Design review of the part built by this model. Coordinates are the model's own, in mm. A direction names the side the tool comes from. Coordinates: 2 decimals unless noted, no trailing zeros. Write each loop counter-clockwise with the first axis right and the second up, starting at its lowest first coordinate (ties: lowest second). Pieces come first, ordered by that corner, then holes. Notation, with made-up numbers: (5, -33.75) - (51, -33.75) arc R12 ccw to (51, -10.75) - close; hole circle Ø11 at (-39.5, 3). An arc over 180 degrees is marked (long way). One line per item, written item: value.
Autodesk Inventor part; units mm, degrees
ref_plane "YZ Plane" through (0, 0, 0) normal (1, 0, 0) x (0, 1, 0)
ref_plane "XZ Plane" through (0, 0, 0) normal (0, 1, 0) x (-1, 0, 0)
ref_plane "XY Plane" through (0, 0, 0) normal (0, 0, 1) x (1, 0, 0)
sketch "Sketch1" plane through (0, 0, 0) normal (0, 1, 0) x (-1, 0, 0)
  line L0 (10, -16) -> (-10, -16)
  line L1 (-10, -16) -> (-10, 16)
  line L2 (-10, 16) -> (10, 16)
  line L3 (10, 16) -> (10, -16)
  point P0 (0, 0)
  point P1 (0, -16)
  point P2 (10, 0)
  dimension "d0" = 20
  dimension "d1" = 32
extrude "Extrusion1" add sketch "Sketch1" along normal blind 1.1
sketch "Sketch2" plane through (0, 1.1, 0) normal (0, 1, 0) x (1, 0, 0)
  circle A0 centre (-7.5, -13.5) radius 1.5
  line L0 (-10, -16) -> (10, -16)
  line L1 (-10, 16) -> (-10, -16)
  line L2 (-10, 0) -> (10, 0) construction
  line L3 (0, -16) -> (0, 16)
  circle A1 centre (-7.5, 13.5) radius 1.5
  circle A2 centre (7.5, -13.5) radius 1.5
  circle A3 centre (7.5, 13.5) radius 1.5
  point P0 (0, 0)
  dimension "d4" = 3
  dimension "d5" = 2.5
  dimension "d6" = 2.5
extrude "Extrusion2" cut sketch "Sketch2" against normal through all
sketch "Sketch3" plane through (0, 1.1, 0) normal (0, 1, 0) x (1, 0, 0)
  circle A0 centre (0, -6) radius 9
  line L0 (-10, -16) -> (10, -16)
  point P0 (0, 0)
  dimension "d9" = 18
  dimension "d10" = 10
extrude "Extrusion3" add sketch "Sketch3" along normal blind 5
fillet "Fillet1" radius 0.5 1 edges at (-9, 6.1, 6)
sketch "Sketch4" plane through (0, 0, 0) normal (1, 0, 0) x (0, 1, 0)
  line L0 (1.1, 15) -> (5.6, 15) construction
  line L1 (1.1, 15) -> (1.1, 12) construction
  arc A0 (6.1, 14.5) -> (5.6, 15) centre (5.6, 14.5) ccw
  line L2 (1.1, 15) -> (1.1, 12.0001)
  line L3 (1.1, 15) -> (1.6, 15)
  line L4 (1.1, 15) -> (1.1, 14.5)
  arc A1 (1.6, 15) -> (1.1, 14.5) centre (1.6, 14.5) ccw
  line L5 (6.1, 6) -> (3.5731, 6) construction
  line L6 (6.1, 14.5) -> (6.1, -2.5) construction
  point P0 (0, 0)
  point P1 (1.1, 6)
  dimension "d17" = 0.5
  dimension "d18" = 0.5
revolve "Revolution1" cut sketch "Sketch4" angle 360 about axis through (0, 6.1, 6) along (0, -1, 0)
sketch "Sketch5" plane through (0, 0, 0) normal (1, 0, 0) x (0, 1, 0)
  line L0 (13.274, 6) -> (6.1, 6)
  line L1 (6.1, 14.5) -> (6.1, -2.5)
  arc A0 (6.1, 14.166) -> (6.9626, 13.1755) centre (7.1, 14.166) ccw
  line L2 (13.274, 12.3) -> (13.274, 6)
  line L3 (13.274, 12.3) -> (6.9626, 13.1755)
  line L4 (6.1, 14.166) -> (6.1, 6)
  line L5 (14.9992, 10.319) -> (14.9992, 6)
  line L6 (13.274, 6) -> (14.9992, 6)
  arc A1 (14.9992, 10.319) -> (13.274, 12.3) centre (12.9992, 10.319) ccw
  point P0 (0, 0)
  point P1 (13.274, 10.9657)
  dimension "d20" = 2
  dimension "d21" = 0.334
  dimension "d22" = 7.174
  dimension "d23" = 6.3
  dimension "d35" = 4
revolve "Revolution2" add sketch "Sketch5" angle 360 about axis through (0, 13.274, 6) along (0, -1, 0)
sketch "Sketch6" plane through (0, 0, 0) normal (0, -1, 0) x (1, 0, 0)
  circle A0 centre (0, 6) radius 7.166
  circle A1 centre (0, 6) radius 5 construction
  circle A2 centre (5, 6) radius 0.5
  circle A3 centre (4.3301, 8.5) radius 0.5
  circle A4 centre (2.5, 10.3301) radius 0.5
  circle A5 centre (0, 11) radius 0.5
  circle A6 centre (-2.5, 10.3301) radius 0.5
  circle A7 centre (-4.3301, 8.5) radius 0.5
  circle A8 centre (-5, 6) radius 0.5
  circle A9 centre (-4.3301, 3.5) radius 0.5
  circle A10 centre (-2.5, 1.6699) radius 0.5
  circle A11 centre (0, 1) radius 0.5
  circle A12 centre (2.5, 1.6699) radius 0.5
  circle A13 centre (4.3301, 3.5) radius 0.5
  point P0 (0, 0)
  dimension "d27" = 10
  dimension "d28" = 1
  dimension "d31" = 360
extrude "Extrusion4" add sketch "Sketch6" along normal blind 5 contours A2 | A3 | A7 | A8 | A9 | A13
sketch "Sketch7" plane through (0, 0, 0) normal (0, -1, 0) x (1, 0, 0)
  line L0 (5, -11) -> (-5, -11)
  line L1 (-5, -11) -> (-5, -13.5)
  line L2 (-5, -13.5) -> (5, -13.5)
  line L3 (5, -13.5) -> (5, -11)
  line L4 (-10, -16) -> (10, -16)
  point P0 (0, 0)
  point P1 (0, -13.5)
  dimension "d36" = 10
  dimension "d37" = 2.5
  dimension "d38" = 2.5
extrude "Extrusion5" add sketch "Sketch7" along normal blind 2.5
sketch "Sketch8" plane through (0, -2.5, 0) normal (0, -1, 0) x (1, 0, 0)
  line L0 (4.2, -12.7) -> (3.3, -12.7)
  line L1 (3.3, -12.7) -> (3.3, -11.8)
  line L2 (3.3, -11.8) -> (4.2, -11.8)
  line L3 (4.2, -11.8) -> (4.2, -12.7)
  line L4 (5, -13.5) -> (5, -11)
  line L5 (5, -11) -> (-5, -11)
  line L6 (-5, -11) -> (-5, -13.5)
  line L7 (-5, -13.5) -> (5, -13.5)
  line L8 (5, -13.5) -> (5, -11)
  line L9 (1.7, -12.7) -> (0.8, -12.7)
  line L10 (1.7, -11.8) -> (1.7, -12.7)
  line L11 (0.8, -12.7) -> (0.8, -11.8)
  line L12 (0.8, -11.8) -> (1.7, -11.8)
  line L13 (-0.8, -12.7) -> (-1.7, -12.7)
  line L14 (-0.8, -11.8) -> (-0.8, -12.7)
  line L15 (-1.7, -12.7) -> (-1.7, -11.8)
  line L16 (-1.7, -11.8) -> (-0.8, -11.8)
  line L17 (-3.3, -12.7) -> (-4.2, -12.7)
  line L18 (-3.3, -11.8) -> (-3.3, -12.7)
  line L19 (-4.2, -12.7) -> (-4.2, -11.8)
  line L20 (-4.2, -11.8) -> (-3.3, -11.8)
  point P0 (0, 0)
  point P1 (5, -12.25)
  point P2 (4.2, -12.25)
  point P3 (1.7, -12.25)
  point P4 (-0.8, -12.25)
  point P5 (-3.3, -12.25)
  dimension "d41" = 0.9
  dimension "d42" = 0.9
  dimension "d43" = 0.8
  dimension "d46" = 2.5
extrude "Extrusion6" add sketch "Sketch8" along normal blind 2 contours L0 L1 L2 L3 | L9 L11 L12 L10 | L13 L15 L16 L14 | L17 L19 L20 L18
sketch "Sketch9" plane through (4.2, -2.5, -12.7) normal (0, 0, -1) x (-1, 0, 0)
  line L0 (0, 0) -> (0.9, 0)
  line L1 (0, 0) -> (0, -2)
  line L2 (0.9, -2) -> (0, -2)
  line L3 (0.9, 0) -> (0.9, -2)
  line L4 (0.9, -1.1) -> (0, -1.1)
  point P0 (4.2, 2.5)
  dimension "d53" = 0.9
  dimension "d54" = 0.9
extrude "Extrusion7" add sketch "Sketch9" along normal blind 8 contours L4 L3 L2 L1
chamfer "Chamfer1" distance 0.3 angle 45 4 edges at (4.2, -4.05, -20.7) (3.75, -4.5, -20.7) (3.3, -4.05, -20.7) (3.75, -3.6, -20.7)
pattern_linear "Rectangular Pattern1" count 4 spacing 2.5 along (-1, 0, 0) of "Extrusion7", "Chamfer1"
equation "\"d53\" = d54"
properties part number "MQ_New" material "Steel, Mild, Welded"
1. Insertion check: pin 1 Ø6 at (y, z) = (5, -7) entering from +X; pin 2 Ø2 at (y, z) = (-3.5, -15) entering from +X; pin 3 Ø4 at (x, y) = (7, 1.5) entering from -Z; pin 4 Ø0.7 at (x, y) = (3.5, -3) entering from -Z. Each pin has a flat end and moves straight along its axis. Give the tip position at first contact, or say it passes through.
Answer block:
pin 1: passes through
pin 2: stops at x = 4.2
pin 3: stops at z = -16
pin 4: stops at z = -12.7
2. For faces 1 (the face through (0, -1, -13.5)), 2 (the face through (-1, -3, -11.8)), 3 (the face through (4.3, -2.5, 3)), 4 (the face through (-5, -1, -12)), 5 (the face through (5, -1, -12)), list the 3-axis set-ups (+Z, -Z, +X, -X, +Y, -Y) from which the entire face can be reached by the end or side of a thin tool; tool diameter is ignored.
Answer block:
face 1: -Z, +X, -X
face 2: +Z, +X, -X, -Y
face 3: -Y
face 4: -Z, -X, -Y
face 5: -Z, +X, -Y
3. Consider section B-B, the plane z = -17.5. Write out the cut boundary in (x, y).
Answer block:
outline: (-4.2, -4.5) - (-3.3, -4.5) - (-3.3, -3.6) - (-4.2, -3.6) - close; (-1.7, -4.5) - (-0.8, -4.5) - (-0.8, -3.6) - (-1.7, -3.6) - close; (0.8, -4.5) - (1.7, -4.5) - (1.7, -3.6) - (0.8, -3.6) - close; (3.3, -4.5) - (4.2, -4.5) - (4.2, -3.6) - (3.3, -3.6) - close
4. Consider section D-D, the plane y = 4. Write out the cut boundary in (x, z).
Answer block:
outline: circle Ø18 at (0, 6)
5. Wall thickness on line 1 along X through (y, z) = (0.4, -13.5); line 2 along Z through (x, y) = (7.5, 0.35); line 3 along Z through (x, y) = (6.25, 1): over which ranges is each line inside the solid? List them lowest first.
Answer block:
line 1: x = -10 to -9, -6 to 6, 9 to 10
line 2: z = -16 to -15, -12 to 12, 15 to 16
line 3: z = -16 to -14.33, -12.67 to 12.67, 14.33 to 16
6. Mouldability with a two-part tool opening along X and no side actions: class faces 6 (the face through (0, -1, -11)), 7 (the face through (-2, 10.78, 12.34)), 8 (the face through (1.7, -4, -16)) as released by +X, released by -X, zero draft, split by the parting line, or undercut.
Answer block:
face 6: zero draft
face 7: split by the parting line
face 8: undercut
7. Consider section A-A, the plane y = 0.5. Write out the cut boundary in (x, z), then the cut area to 3 significant figures.
Answer block:
outline: (-10, -16) - (10, -16) - (10, 16) - (-10, 16) - close; hole circle Ø3 at (-7.5, -13.5); hole circle Ø3 at (-7.5, 13.5); hole circle Ø3 at (7.5, -13.5); hole circle Ø3 at (7.5, 13.5)
area: 612 mm^2
8. Consider section C-C, the plane z = 6. Write out the cut boundary in (x, y), then the cut area to 3 significant figures.
Answer block:
outline: (-10, 0) - (-5.5, 0) - (-5.5, -5) - (-4.5, -5) - (-4.5, 0) - (4.5, 0) - (4.5, -5) - (5.5, -5) - (5.5, 0) - (10, 0) - (10, 1.1) - (8.5, 1.1) arc R0.5 ccw to (9, 1.6) - (9, 5.6) arc R0.5 ccw to (8.5, 6.1) - (8.17, 6.1) arc R1 cw to (7.18, 6.96) - (6.3, 13.27) arc R2 ccw to (4.32, 15) - (-4.32, 15) arc R2 ccw to (-6.3, 13.27) - (-7.18, 6.96) arc R1 cw to (-8.17, 6.1) - (-8.5, 6.1) arc R0.5 ccw to (-9, 5.6) - (-9, 1.6) arc R0.5 ccw to (-8.5, 1.1) - (-10, 1.1) - close
area: 240 mm^2
